from build123d import *

# Parameters (mm, degrees)
BOSS_EXTRUDE12_DEPTH    = 26.67
BOSS_EXTRUDE13_DEPTH    = 2.54
FILLET2_R               = 2.54
SKETCH5_R               = 1.905
CUT_EXTRUDE1_DEPTH      = 58.15
CUT_EXTRUDE1_DEPTH_BACK = 1


with BuildPart() as part:
    # Sketch3 → Boss-Extrude12 (new body)
    with BuildSketch(Plane(origin=(0, 0, 0), x_dir=(1, 0, 0), z_dir=(0, 1, 0))):
        with BuildLine():
            Line((28.575, 13.081), (28.575, 0))
            Line((28.575, 0), (32.893, 0))
            Line((32.893, 0), (32.893, 10.953386454))
            ThreePointArc((32.893, 10.953386454), (49.815156756, 31.75), (32.893, 52.546613546))
            Line((32.893, 52.546613546), (32.893, 63.5))
            Line((32.893, 63.5), (28.575, 63.5))
            Line((28.575, 63.5), (28.575, 50.419))
            ThreePointArc((28.575, 50.419), (41.775976498, 44.950976498), (47.244, 31.75))
            ThreePointArc((47.244, 31.75), (41.775976498, 18.549023502), (28.575, 13.081))
        make_face()
    extrude(amount=BOSS_EXTRUDE12_DEPTH)

    # Sketch3_16 → Boss-Extrude13 (add)
    with BuildSketch(Plane(origin=(0, 0, 0), x_dir=(1, 0, 0), z_dir=(0, 1, 0))):
        with BuildLine():
            Line((32.893, 10.953386454), (32.893, 0))
            Line((32.893, 0), (57.15, 0))
            Line((57.15, 0), (57.15, 63.5))
            Line((57.15, 63.5), (32.893, 63.5))
            Line((32.893, 63.5), (32.893, 52.546613546))
            ThreePointArc((32.893, 52.546613546), (49.815156756, 31.75), (32.893, 10.953386454))
        make_face()
    extrude(amount=BOSS_EXTRUDE13_DEPTH)

    # Fillet2
    fillet2_edges = [part.edges().sort_by_distance(p)[0] for p in [
        (49.815156756, 2.54, -31.75),
        (32.893, 2.54, -5.476693227),
        (32.893, 2.54, -58.023306773),
    ]]
    fillet(fillet2_edges, radius=FILLET2_R)

    # Sketch5 → Cut-Extrude1 (cut, two sides)
    with BuildSketch(Plane(origin=(0, 0, 0), x_dir=(0, 0, -1), z_dir=(1, 0, 0))) as cut_extrude1_sk:
        with Locations((6.5405, 15.24)):
            Circle(SKETCH5_R)
        with Locations((56.41762459, 15.24)):
            Circle(SKETCH5_R)
    extrude(amount=CUT_EXTRUDE1_DEPTH, mode=Mode.SUBTRACT)
    extrude(cut_extrude1_sk.sketch, amount=-CUT_EXTRUDE1_DEPTH_BACK, mode=Mode.SUBTRACT)


solid = part.part
The listing builds one solid part. Answer for the finished solid, in the listing's coordinates (mm). A direction names the side the tool comes from. Coordinates: 2 decimals unless noted, no trailing zeros. Write each loop counter-clockwise with the first axis right and the second up, starting at its lowest first coordinate (ties: lowest second). Pieces come first, ordered by that corner, then holes. Notation, with made-up numbers: (-25, 8) - (17, 8) arc R25 ccw to (17, 45) - close; hole circle Ø9 at (-26, 73.5). An arc over 180 degrees is marked (long way). Put each result on its own line as item: value.
1. A tool of negligible diameter and unlimited length cuts with its end or side. For faces 5 (the face through (32.893, 16, -59)), 6 (the face through (32.893, 16, -4)), 7 (the face through (49.81, 15.72, -31.34)), 8 (the face through (28.575, 13, -57)), 9 (the face through (57.15, 1, -31)), from which of +Z, -Z, +X, -X, +Y, -Y can it reach the whole face along a straight path? Write none if from no direction.
Answer sheet:
face 5: -Z, +X, +Y
face 6: +Z, +X, +Y
face 7: +X, +Y
face 8: +Z, -Z, -X, +Y, -Y
face 9: +Z, -Z, +X, +Y, -Y
2. The part is cut by section A-A on y = 15.24. State how many separate pieces and enclosed holes the cut face has, plus the area to 3 significant figures.
Answer sheet:
separate pieces: 3
enclosed holes: 0
area: 220 mm^2
3. The part is cut by section C-C on x = 55.5. Give the vertices of the cut face in (y, z), plus the area to 3 significant figures.
Answer sheet:
outline: (0, -63.5) - (2.54, -63.5) - (2.54, 0) - (0, 0) - close
area: 161 mm^2
4. Find the intervals of material crossed by line 1 along Z through (x, y) = (31.1, 15.24); line 2 along X through (y, z) = (25.75, -7) (3 decimals); line 3 along Z through (x, y) = (36.25, 4.5), in increasing order. Write a range as from..to.
Answer sheet:
line 1: z = -63.5..-58.32, -54.51..-50.25, -13.25..-8.45, -4.64..0
line 2: x = 28.575..32.893
line 3: z = -51.63..-48.77, -14.73..-11.87
5. Flat-ended cylindrical pins translate along their axes: pin 1 Ø3.5 at (y, z) = (15.24, -6.54) entering from +X; pin 2 Ø3 at (x, y) = (47.5, 17) entering from +Z; pin 3 Ø10 at (y, z) = (22.5, -25.5) entering from -X; pin 4 Ø3 at (y, z) = (20.5, -24.5) entering from +X. Find the tip coordinate at first contact, or state that the pin passes through.
Answer sheet:
pin 1: passes through
pin 2: stops at z = -19.6
pin 3: stops at x = 43.47
pin 4: stops at x = 49.02
6. The part is cut by section B-B on z = -5.5. Give the vertices of the cut face in (x, y) (3 decimals), plus the area to 3 significant figures.
Answer sheet:
outline: (28.575, 0) - (57.15, 0) - (57.15, 2.54) - (35.433, 2.54) arc R2.54 cw to (32.893, 5.08) - (32.893, 13.644) - (28.575, 13.644) - close; (28.575, 16.836) - (32.893, 16.836) - (32.893, 26.67) - (28.575, 26.67) - close
area: 164 mm^2
7. Determine the mould class of faces 1 (the face through (48, 26.67, -32)), 2 (the face through (49, 0, -32)), 3 (the face through (30.7, 13.38, -6.13)), 4 (the face through (32, 8, 0)) for opening direction Y: pulls with the +Y half, pulls with the -Y half, needs draft (parallel to the pull), parting line crosses it, or undercut.
Answer sheet:
face 1: pulls with the +Y half
face 2: pulls with the -Y half
face 3: undercut
face 4: needs draft
